Autodesk Inventor part; units mm, degrees
ref_plane "YZ Plane" through (0, 0, 0) normal (1, 0, 0) x (0, 1, 0)
ref_plane "XZ Plane" through (0, 0, 0) normal (0, 1, 0) x (-1, 0, 0)
ref_plane "XY Plane" through (0, 0, 0) normal (0, 0, 1) x (1, 0, 0)
sketch "Sketch1" plane through (0, 0, 0) normal (0, 0, 1) x (1, 0, 0)
  circle A0 centre (0, 0) radius 37.5
  dimension "d0" = 75
extrude "Extrusion1" add sketch "Sketch1" along normal blind 40
sketch "Sketch2" plane through (0, 0, 0) normal (0, 0, -1) x (-1, 0, 0)
  circle A0 centre (0, 0) radius 30
  circle A1 centre (-1.5403, 0) radius 25
  dimension "d3" = 60
  dimension "d4" = 50
extrude "Extrusion2" add sketch "Sketch2" along normal blind 20
sketch "Sketch3" plane through (0, 0, 0) normal (1, 0, 0) x (0, 1, 0)
  line L0 (37.5, 40) -> (-37.5, 40)
  line L1 (20, 40) -> (58.4777, 40)
  line L2 (20, 190) -> (20, 40)
  line L3 (58.4777, 40) -> (36.0386, 174.5807)
  line L4 (36.0386, 174.5807) -> (20, 190)
  line L5 (0, 40) -> (0, 219.4049)
  line L6 (-20, 40) -> (-58.4777, 40)
  line L7 (-20, 190) -> (-20, 40)
  line L8 (-58.4777, 40) -> (-36.0386, 174.5807)
  line L9 (-36.0386, 174.5807) -> (-20, 190)
  point P0 (0, 0)
  dimension "d8" = 150
  dimension "d11" = 40
extrude "Extrusion3" add sketch "Sketch3" along normal mid plane 10
properties part number "Grip"
For this review, take the finished solid that the model builds, in its own axes (mm). A direction names the side the tool comes from. Coordinates: 2 decimals unless noted, no trailing zeros. Order: outer loops, then holes, each group sorted by start corner. A loop starts at its lowest first (then second) coordinate and runs counter-clockwise, first axis right, second up. Notation, with made-up numbers: (28, 60.5) -> (69, 60.5) arc R33 ccw to (69, 92.5) -> close; hole circle Ø2 at (37.25, -17). An arc over 180 degrees is marked (long way). Return JSON: item names as keys, results as strings.
1. The part is to be moulded in two halves that separate along X. For faces 1 (the flat face through (-0.07, -28.132, 182.182)), 2 (the cylindrical face through (-4.88, -37.18, 19.72)), 3 (the flat face through (1, 0, 0)), say which applies: +X half, -X half, draft (parallel to the pull), parting line (faces both ways), or undercut.
Answer block:
{"face 1": "draft", "face 2": "parting line", "face 3": "undercut"}
2. Machinability: for faces 4 (the flat face through (-5, -35, 99)), 5 (the flat face through (-17, 25, 0)), 6 (the flat face through (0, 20, 116)), which of the approach directions +Z, -Z, +X, -X, +Y, -Y give a long, thin tool a straight path to every point of the face, cutting with its end or side? Answer none if there is none.
Answer block:
{"face 4": "+Z, -X, +Y, -Y", "face 5": "-Z", "face 6": "+Z, +X, -X"}
3. We need section A-A on z = 124. Write out the cut boundary in (x, y).
Answer block:
{"outline": "(-5, -44.47) -> (5, -44.47) -> (5, -20) -> (-5, -20) -> close; (-5, 20) -> (5, 20) -> (5, 44.47) -> (-5, 44.47) -> close"}
4. We need section C-C on x = 10. Write out the cut boundary in (y, z).
Answer block:
{"outline": "(-36.14, 0) -> (-28.28, 0) -> (-28.28, -20) -> (-23.53, -20) -> (-23.53, 0) -> (23.53, 0) -> (23.53, -20) -> (28.28, -20) -> (28.28, 0) -> (36.14, 0) -> (36.14, 40) -> (-36.14, 40) -> close"}
5. We need section D-D on z = -4. Write out the cut boundary in (x, y).
Answer block:
{"outline": "circle Ø60 at (0, 0); hole circle Ø50 at (1.54, 0)"}
6. For line 1 (Z direction, x = 13.5, y = 3.5); line 2 (X direction, y = -21, z = 119.5); line 3 (Y direction, x = 4.5, z = 89.5), list the stretches that pass through material, from the lowest coordinate up. Write a range as from..to.
Answer block:
{"line 1": "0..40", "line 2": "-5..5", "line 3": "-50.22..-20, 20..50.22"}
7. For pin 1 Ø19 at (y, z) = (-36, 80) entering from -X; pin 2 Ø5 at (x, z) = (-0.5, 131.5) entering from +Y; pin 3 Ø8 at (x, z) = (-0.5, 110.5) entering from -Y, all flat-tipped, find the tip position at first contact; note any pin that passes through.
Answer block:
{"pin 1": "x = -5", "pin 2": "y = 43.64", "pin 3": "y = -47.39"}
8. We need section B-B on y = 0. Write out the cut boundary in (x, z), and give its area (3 significant figures).
Answer block:
{"outline": "(-37.5, 0) -> (-30, 0) -> (-30, -20) -> (-23.46, -20) -> (-23.46, 0) -> (26.54, 0) -> (26.54, -20) -> (30, -20) -> (30, 0) -> (37.5, 0) -> (37.5, 40) -> (-37.5, 40) -> close", "area": "3,200 mm²"}
